For this review, take the finished solid that the model builds, in its own axes (mm). Face numbers are marked on the shaded views. A direction names the side the tool comes from. Coordinates: 2 decimals unless noted, no trailing zeros. Loops run counter-clockwise (first coordinate to the right, second up) from the corner with the lowest first, then second, coordinate; pieces in that order, holes last. Notation, with made-up numbers: M 12.25,87.5 L 47.25,87.5 A29 ccw 47.25,119.5 Z; hole C -22.75,46 d11. An arc over 180 degrees is marked long. Put each result on its own line as item: value.
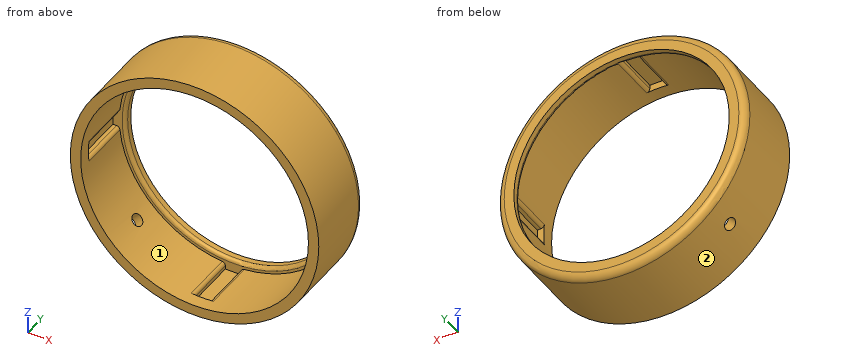
```python
from build123d import *

# Parameters (mm, degrees)
SKETCH1_R                       = 45.72
BOSS_EXTRUDE1_DEPTH             = 22.225
SKETCH6_R                       = 39.624
CUT_EXTRUDE1_DEPTH              = 23.225
SKETCH8_R                       = 41.91
CUT_EXTRUDE2_DEPTH              = 19.05
FILLET1_R                       = 2.54
F_17_0_173_DIAMETER_HOLE2_D     = 4.3942
F_17_0_173_DIAMETER_HOLE2_DEPTH = 22.745829939
SKETCH25_W                      = 88.646
SKETCH25_H                      = 5.842
CUT_EXTRUDE7_DEPTH              = 19.05
SKETCH27_W                      = 5.842
SKETCH27_H                      = 88.646
CUT_EXTRUDE8_DEPTH              = 19.05
FILLET2_R                       = 1.27
FILLET3_R                       = 1.27
SKETCH36_R                      = 45.72
BOSS_EXTRUDE4_DEPTH             = 4.7625
SKETCH37_R                      = 41.91
CUT_EXTRUDE11_DEPTH             = 4.7625


with BuildPart() as part:
    # Sketch1 → Boss-Extrude1 (new body)
    with BuildSketch(Plane(origin=(0, 0, 0), x_dir=(1, 0, 0), z_dir=(0, 1, 0))):
        Circle(SKETCH1_R)
    extrude(amount=BOSS_EXTRUDE1_DEPTH)

    # Sketch6 → Cut-Extrude1 (cut, through all)
    with BuildSketch(Plane(origin=(0, 22.225, 0), x_dir=(1, 0, 0), z_dir=(0, 1, 0))):
        Circle(SKETCH6_R)
    extrude(amount=-CUT_EXTRUDE1_DEPTH, mode=Mode.SUBTRACT)

    # Sketch8 → Cut-Extrude2 (cut)
    with BuildSketch(Plane.XZ):
        Circle(SKETCH8_R)
    extrude(amount=-CUT_EXTRUDE2_DEPTH, mode=Mode.SUBTRACT)

    # Fillet1
    fillet1_edges = [part.edges().sort_by_distance(p)[0] for p in [
        (-45.72, 22.225, 0),
    ]]
    fillet(fillet1_edges, radius=FILLET1_R)

    # #17 (0.173) Diameter Hole2
    with Locations(Plane(origin=(-29.867831461, 9.910321026, -29.40001265), x_dir=(-0.701503523, 0, 0.712665986), z_dir=(0.712665986, 0, 0.701503523))):
        with Locations((0, 0)):
            Hole(F_17_0_173_DIAMETER_HOLE2_D / 2, depth=F_17_0_173_DIAMETER_HOLE2_DEPTH)

    # Sketch25 → Cut-Extrude7 (cut)
    with BuildSketch(Plane.XZ):
        Rectangle(SKETCH25_W, SKETCH25_H)
    extrude(amount=-CUT_EXTRUDE7_DEPTH, mode=Mode.SUBTRACT)

    # Sketch27 → Cut-Extrude8 (cut)
    with BuildSketch(Plane.XZ):
        Rectangle(SKETCH27_W, SKETCH27_H)
    extrude(amount=-CUT_EXTRUDE8_DEPTH, mode=Mode.SUBTRACT)

    # Fillet2
    fillet2_edges = [part.edges().sort_by_distance(p)[0] for p in [
        (41.808083656, 9.525, 2.921),
        (-41.808083656, 9.525, 2.921),
        (41.808083656, 9.525, -2.921),
        (-41.808083656, 9.525, -2.921),
        (2.921, 9.525, 41.808083656),
        (-2.921, 9.525, 41.808083656),
        (-2.921, 9.525, -41.808083656),
        (2.921, 9.525, -41.808083656),
    ]]
    fillet(fillet2_edges, radius=FILLET2_R)

    # Fillet3
    fillet3_edges = [part.edges().sort_by_distance(p)[0] for p in [
        (-39.624, 19.05, 0),
    ]]
    fillet(fillet3_edges, radius=FILLET3_R)

    # Sketch36 → Boss-Extrude4 (add)
    with BuildSketch(Plane.XZ):
        Circle(SKETCH36_R)
    extrude(amount=BOSS_EXTRUDE4_DEPTH)

    # Sketch37 → Cut-Extrude11 (cut)
    with BuildSketch(Plane(origin=(0, 0, 0), x_dir=(1, 0, 0), z_dir=(0, 1, 0))):
        Circle(SKETCH37_R)
    extrude(amount=-CUT_EXTRUDE11_DEPTH, mode=Mode.SUBTRACT)


solid = part.part
```
(1) Wall thickness on line 1 along X through (y, z) = (4, 0); line 2 along Z through (x, y) = (19.5, 5.75); line 3 along X through (y, z) = (21.85, 0): over which ranges is each line inside the solid? List them lowest first. Write a range as [from, to].
Determined:
line 1: x = [-45.72, -44.32], [44.32, 45.72]
line 2: z = [-41.35, -37.1], [37.1, 41.35]
line 3: x = [-44.51, -39.62], [39.62, 44.51]
(2) For pin 1 (1.5 mm diameter, centred on y = 5, z = -25.5, fed in from -X); pin 2 (2 mm diameter, centred on x = -11, y = 3.5, fed in from -Z); pin 3 (10 mm diameter, centred on y = 1.5, z = -17, fed in from +X), all flat-tipped, find the tip position at first contact; note any pin that passes through.
Determined:
pin 1: stops at x = -38.44
pin 2: stops at z = -44.61
pin 3: stops at x = 44.12
(3) Add section C-C (y = 2.75). Write out the cut boundary in (x, z), plus the area to 3 significant figures.
Determined:
outline: C 0,0 d91.44; hole M -44.32,-2.92 L -42.98,-2.92 A1.27 cw -41.71,-4.07 A41.91 ccw -4.07,-41.71 A1.27 cw -2.92,-42.98 L -2.92,-44.32 L 2.92,-44.32 L 2.92,-42.98 A1.27 cw 4.07,-41.71 A41.91 ccw 41.71,-4.07 A1.27 cw 42.98,-2.92 L 44.32,-2.92 L 44.32,2.92 L 42.98,2.92 A1.27 cw 41.71,4.07 A41.91 ccw 4.07,41.71 A1.27 cw 2.92,42.98 L 2.92,44.32 L -2.92,44.32 L -2.92,42.98 A1.27 cw -4.07,41.71 A41.91 ccw -41.71,4.07 A1.27 cw -42.98,2.92 L -44.32,2.92 Z
area: 989 mm^2
(4) Tool access review of the marked faces 1 and 2: name each direction out of +Z, -Z, +X, -X, +Y, -Y from which nothing blocks a thin tool from reaching the whole face with its end or side.
Determined:
face 1: -Y
face 2: +Y, -Y
